Model file for the job. Use its own axes, mm. Face numbers are marked on the shaded views. A direction names the side the tool comes from. Give positions to 0.01 mm unless a question says otherwise; leave off trailing zeros. Write each loop counter-clockwise with the first axis right and the second up, starting at its lowest first coordinate (ties: lowest second). Pieces come first, ordered by that corner, then holes.
```python
from build123d import *

# Parameters (mm, degrees)
SKETCH225_R     = 1.5
PAD127060_DEPTH = 100
SKETCH223_R     = 1.8
SKETCH223_W     = 2.5
SKETCH223_H     = 13
PAD127058_DEPTH = 3
SKETCH224_W     = 44
SKETCH224_H     = 23
PAD127059_DEPTH = 15


with BuildPart() as mountingscrewcutouts:
    # Sketch225 → Pad127060 (new body)
    with BuildSketch(Plane(origin=(50, 160, 11.5), x_dir=(1, 0, 0), z_dir=(0, 0, 1))):
        with Locations((-32, -63)):
            Circle(SKETCH225_R)
        with Locations((-42, -63)):
            Circle(SKETCH225_R)
        with Locations((-32, -56)):
            Circle(SKETCH225_R)
        with Locations((-42, -56)):
            Circle(SKETCH225_R)
    extrude(amount=-PAD127060_DEPTH)


with BuildPart() as cutouts:
    # Part__Mirroring016: instance of MountingScrewCutouts
    add(mountingscrewcutouts.part.mirror(Plane(origin=(0, 0, 0), x_dir=(0, -1, 0), z_dir=(1, 0, 0))))

    # Fusion004020033: union MountingScrewCutouts
    add(mountingscrewcutouts.part)


with BuildPart() as baseplate:
    # Sketch223 → Pad127058 (new body)
    with BuildSketch(Plane.XZ.offset(-93)):
        with BuildLine():
            Line((-29.490381, 15), (-39.5, 9.220944))
            Line((-39.5, 9.220944), (-39.5, -9.220944))
            Line((-39.5, -9.220944), (-29.490381, -15))
            Line((-23.428203, -11.5), (-29.490381, -15))
            Line((-23.428203, -11.5), (0, -11.5))
            Line((0, -8), (0, -11.5))
            Line((0, -8), (-12, -8))
            ThreePointArc((-12, 8), (-20, 0), (-12, -8))
            Line((0, 8), (-12, 8))
            Line((0, 11.5), (0, 8))
            Line((-23.428203, 11.5), (0, 11.5))
            Line((-29.490381, 15), (-23.428203, 11.5))
        make_face()
        with Locations((-29, 10)):
            Circle(SKETCH223_R, mode=Mode.SUBTRACT)
        with Locations((-29, -10)):
            Circle(SKETCH223_R, mode=Mode.SUBTRACT)
        with Locations((-36, 0)):
            Circle(SKETCH223_R, mode=Mode.SUBTRACT)
        with Locations((-30.25, 0)):
            Rectangle(SKETCH223_W, SKETCH223_H, mode=Mode.SUBTRACT)
    extrude(amount=-PAD127058_DEPTH)


with BuildPart() as mountingblock:
    # Sketch224 → Pad127059 (new body)
    with BuildSketch(Plane.XZ.offset(-93)):
        Rectangle(SKETCH224_W, SKETCH224_H)
        with BuildLine():
            ThreePointArc((-12, 8), (-20, 0), (-12, -8))
            Line((-12, -8), (12, -8))
            ThreePointArc((12, -8), (20, 0), (12, 8))
            Line((-12, 8), (12, 8))
        make_face(mode=Mode.SUBTRACT)
    extrude(amount=-PAD127059_DEPTH)


with BuildPart() as interfaceblock:
    # Part__Mirroring015: instance of BasePlate
    add(baseplate.part.mirror(Plane(origin=(0, 0, 0), x_dir=(0, -1, 0), z_dir=(1, 0, 0))))

    # Fusion004020032: union BasePlate, MountingBlock
    add(baseplate.part)
    add(mountingblock.part)

    # Cut007019030: cut Cutouts
    add(cutouts.part, mode=Mode.SUBTRACT)


solid = interfaceblock.part
```
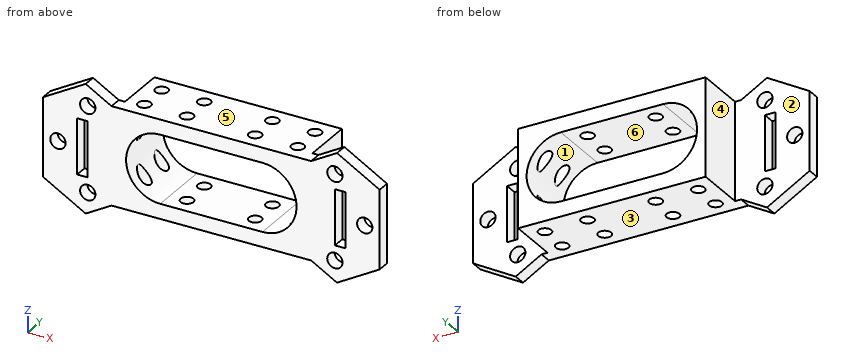
1. Probe probe 1 along X at (y, z) = (97, -9.15); probe 2 along Z at (x, y) = (-12, 107); probe 3 along Z at (x, y) = (-16.5, 97.75). List the from-to ranges inside material, lowest first.
Calculated:
probe 1: x = -22 to -19.5, -16.5 to -9.5, -6.5 to 6.5, 9.5 to 16.5, 19.5 to 22
probe 2: z = -11.5 to -8, 8 to 11.5
probe 3: z = -11.5 to -6.61, 6.61 to 11.5
2. Slice it at B-B, the plane z = 0. Write the cut outline in (x, y), and give its area (3 significant figures).
Calculated:
outline: (-39.5, 93) - (-37.8, 93) - (-37.8, 96) - (-39.5, 96) - close; (-34.2, 93) - (-31.5, 93) - (-31.5, 96) - (-34.2, 96) - close; (-29, 93) - (-20, 93) - (-20, 108) - (-22, 108) - (-22, 96) - (-29, 96) - close; (20, 93) - (29, 93) - (29, 96) - (22, 96) - (22, 108) - (20, 108) - close; (31.5, 93) - (34.2, 93) - (34.2, 96) - (31.5, 96) - close; (37.8, 93) - (39.5, 93) - (39.5, 96) - (37.8, 96) - close
area: 128 mm2
3. Pin check, flat tips, straight feed: P1, Ø3.5, axis at y = 99, z = -3, coming from the +X side; P2, Ø5, axis at x = -7.5, y = 102.5, coming from the -Z side; P3, Ø1.2, axis at x = -30.5, y = 94, coming from the -Z side. Stop position of each tip, or through.
Calculated:
P1: stops at x = 22
P2: stops at z = -11.5
P3: stops at z = -14.76
4. Pull direction Z, two halves, no side cores. Call the marked faces 4, 5 and 6: +Z half, -Z half, draft (parallel to the pull), parting line (faces both ways), or undercut.
Calculated:
face 4: draft
face 5: +Z half
face 6: undercut
5. Slice it at C-C, the plane y = 94.5. State how many separate pieces and enclosed holes the cut face has, and give its area (3 significant figures).
Calculated:
separate pieces: 1
enclosed holes: 9
area: 1,170 mm2
6. Slice it at D-D, the plane z = 7.25. Write the cut outline in (x, y).
Calculated:
outline: (-39.5, 93) - (-15.38, 93) - (-15.38, 108) - (-22, 108) - (-22, 96) - (-39.5, 96) - close; (15.38, 93) - (39.5, 93) - (39.5, 96) - (22, 96) - (22, 108) - (15.38, 108) - close; hole circle Ø3 at (-18, 97); hole circle Ø3 at (-18, 104); hole circle Ø3 at (18, 97); hole circle Ø3 at (18, 104)
7. Slice it at A-A, the plane x = -8. Write the cut outline in (y, z).
Calculated:
outline: (93, -11.5) - (95.5, -11.5) - (95.5, -8) - (93, -8) - close; (93, 8) - (95.5, 8) - (95.5, 11.5) - (93, 11.5) - close; (98.5, -11.5) - (102.5, -11.5) - (102.5, -8) - (98.5, -8) - close; (98.5, 8) - (102.5, 8) - (102.5, 11.5) - (98.5, 11.5) - close; (105.5, -11.5) - (108, -11.5) - (108, -8) - (105.5, -8) - close; (105.5, 8) - (108, 8) - (108, 11.5) - (105.5, 11.5) - close
8. Which spindle directions (+Z, -Z, +X, -X, +Y, -Y) get a long thin tool onto all of the face, cutting with end or side? Do the marked faces 1, 2 and 3. Say none if no direction does.
Calculated:
face 1: +Y, -Y
face 2: +Z, -Z, -X, +Y
face 3: -Z, +Y, -Y
